Part model, mm, in its own coordinate system. A direction names the side the tool comes from. Give positions to 0.01 mm unless a question says otherwise; leave off trailing zeros. Write each loop counter-clockwise with the first axis right and the second up, starting at its lowest first coordinate (ties: lowest second). Pieces come first, ordered by that corner, then holes. Notation, with made-up numbers: M 39.5,48.5 L 71.5,48.5 A15 ccw 71.5,53.5 Z; hole C 17.25,26.5 d7. An arc over 180 degrees is marked long. Use CSV: the item, a comma, the result in double quotes. Start each with the question number.
1. Mould opens along X. For faces 1 (the face through (0, 0, -10)), 2 (the face through (19.715, 19.699, -0.126)), 3 (the face through (-17, 15, 0)) say: pulls with the +X half, pulls with the -X half, needs draft (parallel to the pull), parting line crosses it, or undercut.
2. Drill centre lines: line 1 along X through (y, z) = (-16.6, -7.5); line 2 along X through (y, z) = (17.3, 0) (3 decimals); line 3 along Y through (x, z) = (-7, 7.25). Where is each one in solid material? Low to high. Write a range as from..to.
3. Band-saw the part on A-A, the plane x = -10. List the corners of the cut face in (y, z), then the cut area to 3 significant figures.
4. 3-axis set-ups, long thin cutter, end or side, ignore diameter. For faces 4 (the face through (11.735, -22.249, 0.228)), 5 (the face through (13, 18, -0.4)), 6 (the face through (0.266, 19.699, 9.715)): which of +Z, -Z, +X, -X, +Y, -Y reach the whole face in a straight line?
5. Drop flat-ended pins along their axis: pin 1 Ø2 at (x, z) = (-2.5, 7.5) entering from +Y; pin 2 Ø1.5 at (x, z) = (15.5, 3) entering from -Y; pin 3 Ø10 at (x, z) = (-3, -7.5) entering from -Y; pin 4 Ø9.5 at (x, z) = (11.5, -0.5) entering from -Y. Give the stop position or say it passes through.
from build123d import *

# Parameters (mm, degrees)
SKETCH_1_W          = 40
SKETCH_1_H          = 40
EXTRUDE_1_DEPTH     = 10
FILLET_1_R          = 1
SKETCH_5_R          = 0.8
CUT_EXTRUDE_2_DEPTH = 5
SKETCH_6_R          = 0.8
CUT_EXTRUDE_3_DEPTH = 5
SKETCH_2_R          = 6.5
EXTRUDE_2_DEPTH     = 1.5
SKETCH_2_3_R        = 3.75
EXTRUDE_3_DEPTH     = 1.8
SKETCH_2_4_R        = 3
EXTRUDE_4_DEPTH     = 5.7
CUT_EXTRUDE_START   = 5.7
SKETCH_2_5_R        = 1.75
CUT_EXTRUDE_4_DEPTH = 7
FILLET_2_R          = 0.5
EXTRUDE_START       = 1.5
SKETCH_4_R          = 6.5
EXTRUDE_5_DEPTH     = 1.5
CUT_EXTRUDE_START_2 = 1.5
SKETCH_4_4_R        = 3.025
CUT_EXTRUDE_5_DEPTH = 7
FILLET_3_R          = 0.5


with BuildPart() as part:
    # 草图1 → 凸台-拉伸1 (new, symmetric)
    with BuildSketch(Plane.XY):
        Rectangle(SKETCH_1_W, SKETCH_1_H)
    extrude(amount=EXTRUDE_1_DEPTH, both=True)

    # 圆角1
    fillet_1_edges = [part.edges().sort_by_distance(p)[0] for p in [
        (-20, 0, 10),
        (0, -20, 10),
        (20, 0, 10),
        (0, -20, -10),
        (-20, 0, -10),
        (0, 20, -10),
        (20, 0, -10),
        (0, 20, 10),
        (20, -20, 0),
        (-20, -20, 0),
        (-20, 20, 0),
        (20, 20, 0),
    ]]
    fillet(fillet_1_edges, radius=FILLET_1_R)

    # 草图5 → 切除-拉伸2 (cut)
    with BuildSketch(Plane(origin=(0, -20, 0), x_dir=(-1, 0, 0), z_dir=(0, -1, 0))):
        with Locations(Location((17.5, -7.5, 0), (0, 0, 90))):
            Circle(SKETCH_5_R)
        with Locations(Location((2.5, -7.5, 0), (0, 0, 90))):
            Circle(SKETCH_5_R)
        with Locations(Location((2.5, 7.5, 0), (0, 0, 90))):
            Circle(SKETCH_5_R)
        with Locations(Location((17.5, 7.5, 0), (0, 0, 90))):
            Circle(SKETCH_5_R)
    extrude(amount=-CUT_EXTRUDE_2_DEPTH, mode=Mode.SUBTRACT)

    # 草图6 → 切除-拉伸3 (cut)
    with BuildSketch(Plane(origin=(0, 20, 0), x_dir=(1, 0, 0), z_dir=(0, 1, 0))):
        with Locations(Location((-10, 7, 0), (0, 0, 270))):
            Circle(SKETCH_6_R)
        with Locations(Location((-17, 0, 0), (0, 0, 270))):
            Circle(SKETCH_6_R)
        with Locations(Location((-10, -7, 0), (0, 0, 270))):
            Circle(SKETCH_6_R)
    extrude(amount=-CUT_EXTRUDE_3_DEPTH, mode=Mode.SUBTRACT)

    # 草图2 → 凸台-拉伸2 (add)
    with BuildSketch(Plane.XZ.offset(20)):
        with Locations(Location((10, 0, 0), (0, 0, 90))):
            Circle(SKETCH_2_R)
    extrude(amount=EXTRUDE_2_DEPTH)

    # 草图2<3> → 凸台-拉伸3 (add)
    with BuildSketch(Plane.XZ.offset(20)):
        with Locations(Location((10, 0, 0), (0, 0, 270))):
            Circle(SKETCH_2_3_R)
    extrude(amount=EXTRUDE_3_DEPTH)

    # 草图2<4> → 凸台-拉伸4 (add)
    with BuildSketch(Plane.XZ.offset(20)):
        with Locations(Location((10, 0, 0), (0, 0, 270))):
            Circle(SKETCH_2_4_R)
    extrude(amount=EXTRUDE_4_DEPTH)

    # 草图2<5> → 切除-拉伸4 (cut)
    with BuildSketch(Plane.XZ.offset(20).offset(CUT_EXTRUDE_START)):
        with Locations(Location((10, 0, 0), (0, 0, 270))):
            Circle(SKETCH_2_5_R)
    extrude(amount=-CUT_EXTRUDE_4_DEPTH, mode=Mode.SUBTRACT)

    # 圆角2
    fillet_2_edges = [part.edges().sort_by_distance(p)[0] for p in [
        (10, -21.5, -6.5),
    ]]
    fillet(fillet_2_edges, radius=FILLET_2_R)

    # 草图4 → 凸台-拉伸5 (add)
    with BuildSketch(Plane(origin=(0, 20, 0), x_dir=(1, 0, 0), z_dir=(0, 1, 0)).offset(EXTRUDE_START)):
        with Locations(Location((10, 0, 0), (0, 0, 270))):
            Circle(SKETCH_4_R)
    extrude(amount=-EXTRUDE_5_DEPTH)

    # 草图4<4> → 切除-拉伸5 (cut)
    with BuildSketch(Plane(origin=(0, 20, 0), x_dir=(1, 0, 0), z_dir=(0, 1, 0)).offset(CUT_EXTRUDE_START_2)):
        with Locations(Location((10, 0, 0), (0, 0, 270))):
            Circle(SKETCH_4_4_R)
    extrude(amount=-CUT_EXTRUDE_5_DEPTH, mode=Mode.SUBTRACT)

    # 圆角3
    fillet_3_edges = [part.edges().sort_by_distance(p)[0] for p in [
        (10, 21.5, -6.5),
    ]]
    fillet(fillet_3_edges, radius=FILLET_3_R)


solid = part.part
Output:
1,face 1,"needs draft"
1,face 2,"pulls with the +X half"
1,face 3,"undercut"
2,line 1,"x = -20..-18.3, -16.7..-3.3, -1.7..20"
2,line 2,"x = -20..-17.8, -16.2..6.975, 13.025..20"
2,line 3,"y = -20..20"
3,outline,"M -20,-9 A1 ccw -19,-10 L 19,-10 A1 ccw 20,-9 L 20,-7.8 L 15,-7.8 L 15,-6.2 L 20,-6.2 L 20,6.2 L 15,6.2 L 15,7.8 L 20,7.8 L 20,9 A1 ccw 19,10 L -19,10 A1 ccw -20,9 Z"
3,area,"783 mm²"
4,face 4,"-Y"
4,face 5,"+Y"
4,face 6,"+Z, +X, -X, +Y"
5,pin 1,"stops at y = 20"
5,pin 2,"stops at y = -21.5"
5,pin 3,"stops at y = -20"
5,pin 4,"stops at y = -25.7"
